from build123d import *

# Parameters (mm, degrees)
SKETCH_1_W             = 95
SKETCH_1_H             = 95
EXTRUDE_1_DEPTH        = 2
SKETCH_2_W             = 95
SKETCH_2_H             = 2
EXTRUDE_2_DEPTH        = 10
FILLET_1_R             = 20
SKETCH_3_W             = 60
SKETCH_3_H             = 10
CUT_EXTRUDE_1_DEPTH    = 106.115412761
EXTRUDE_START          = 33
EXTRUDE_3_DEPTH        = 1
PATTERN_LINEAR_1_COUNT = 2
PATTERN_LINEAR_1_PITCH = 12
MIRROR_START           = 33
MIRROR_1_COPY_1_DEPTH  = 1
SKETCH_7_R             = 1.5
CUT_EXTRUDE_2_DEPTH    = 2


with BuildPart() as part:
    # 草图1 → 凸台-拉伸1 (new body)
    with BuildSketch(Plane.XY):
        Rectangle(SKETCH_1_W, SKETCH_1_H)
    extrude(amount=EXTRUDE_1_DEPTH)

    # 草图2 → 凸台-拉伸2 (add)
    with BuildSketch(Plane.XY.offset(2)):
        with Locations((0, -46.5)):
            Rectangle(SKETCH_2_W, SKETCH_2_H)
    extrude(amount=EXTRUDE_2_DEPTH)

    # 圆角1
    fillet_1_edges = [part.edges().sort_by_distance(p)[0] for p in [
        (-47.5, 47.5, 1),
        (47.5, 47.5, 1),
    ]]
    fillet(fillet_1_edges, radius=FILLET_1_R)

    # 草图3 → 切除-拉伸1 (cut, through all)
    with BuildSketch(Plane(origin=(0, -45.5, 0), x_dir=(1, 0, 0), z_dir=(0, 1, 0))):
        with Locations((0, -7)):
            Rectangle(SKETCH_3_W, SKETCH_3_H)
    extrude(amount=-CUT_EXTRUDE_1_DEPTH, mode=Mode.SUBTRACT)

    # 草图5 → 凸台-拉伸3 (add, symmetric)
    with BuildSketch(Plane(origin=(0, 0, 0), x_dir=(0, 0, -1), z_dir=(1, 0, 0)).offset(EXTRUDE_START)):
        Polygon((-1.499876111, -46.213636553), (-1.499876111, -21.213636553), (-10.151701689, -46.213636553), align=None)
    extrude_3 = extrude(amount=EXTRUDE_3_DEPTH, both=True)

    # 阵列(线性)1: 凸台-拉伸3 ×2
    with Locations(*[(i * PATTERN_LINEAR_1_PITCH, 0, 0) for i in range(1, PATTERN_LINEAR_1_COUNT)]):
        add(extrude_3)

    # 镜向1: 凸台-拉伸3 across plane
    add(extrude_3.mirror(Plane(origin=(0, 0, 0), x_dir=(0, 0, 1), z_dir=(1, 0, 0))))

    # 镜向1 copy 1 sketch → 镜向1 copy 1 (add, symmetric)
    with BuildSketch(Plane(origin=(-12, 0, 0), x_dir=(0, 0, -1), z_dir=(-1, 0, 0)).offset(MIRROR_START)):
        Polygon((-1.499876111, 46.213636553), (-1.499876111, 21.213636553), (-10.151701689, 46.213636553), align=None)
    extrude(amount=MIRROR_1_COPY_1_DEPTH, both=True)

    # 草图7 → 切除-拉伸2 (cut)
    with BuildSketch(Plane(origin=(0, -45.5, 0), x_dir=(1, 0, 0), z_dir=(0, 1, 0))):
        with Locations(Location((-39, -7, 0), (0, 0, 270))):
            Circle(SKETCH_7_R)
        with Locations(Location((39, -7, 0), (0, 0, 90))):
            Circle(SKETCH_7_R)
    extrude(amount=-CUT_EXTRUDE_2_DEPTH, mode=Mode.SUBTRACT)


solid = part.part
Source: CAD feature listing. Evaluate the final solid. Frame: model axes, mm. A direction names the side the tool comes from. Round coordinates to 2 decimals unless told otherwise and drop trailing zeros. Loops run counter-clockwise (first coordinate to the right, second up) from the corner with the lowest first, then second, coordinate; pieces in that order, holes last.
Q1. Mould query, pull axis X, two halves, no side actions, for faces 1 (the face through (34, -39, 4)), 2 (the face through (-44, -37, 5)), 3 (the face through (47.5, -15.7, 1.5)), 4 (the face through (-33.014, -33.919, 5.897)). Classes: pulls with the +X half, pulls with the -X half, needs draft (parallel to the pull), parting line crosses it, or undercut.
Q2. First-contact query: P1, Ø2, axis at x = 35, y = 36, coming from the +Z side; P2, Ø6.5, axis at y = -32.5, z = 5.5, coming from the -X side; P3, Ø3, axis at x = 39, z = 6.5, coming from the +Y side. Flat tips, straight axial feed; report the tip coordinate or a pass-through.
Q3. Access query for faces 5 (the face through (46, -39, 4)), 6 (the face through (40.464, -46.486, 7.325)), 7 (the face through (-37, -45.5, 7)), 8 (the face through (-41.797, 41.486, 1.014)), 9 (the face through (-46, -37, 5)). Directions: +Z, -Z, +X, -X, +Y, -Y. A direction counts if a zero-diameter tool reaches every point of the face in a straight line with its end or side. Return the directions, or none.
Q4. Section C-C, the plane y = -4. Return loops of the section in (x, z).
Q5. Section A-A, the plane x = 39. Return loops of the section in (y, z).
Q6. Section B-B, the plane z = 7. State how many separate pieces and enclosed holes the cut face has, plus the area to 3 significant figures.
Q7. Ray query, line 1 (X direction, y = -46.2, z = 7); line 2 (X direction, y = -43, z = 7.25); line 3 (Z direction, x = 39, y = -46). Return the intervals inside material, ascending.
Solutions:
1. face 1: undercut
1. face 2: undercut
1. face 3: pulls with the +X half
1. face 4: needs draft
2. P1: stops at z = 2
2. P2: stops at x = -46
2. P3: stops at y = -45.5
3. face 5: +Z, +X, +Y
3. face 6: +Y, -Y
3. face 7: +Z, +Y
3. face 8: +Z, -Z, -X, +Y
3. face 9: +Z, -X, +Y
4. outline: (-47.5, 0) - (47.5, 0) - (47.5, 2) - (-47.5, 2) - close
5. outline: (-47.5, 0) - (43.86, 0) - (43.86, 2) - (-45.5, 2) - (-45.5, 5.5) - (-47.5, 5.5) - close; (-47.5, 8.5) - (-45.5, 8.5) - (-45.5, 12) - (-47.5, 12) - close
6. separate pieces: 4
6. enclosed holes: 0
6. area: 125 mm2
7. line 1: x = -47.5 to -40.5, -37.5 to -30, 30 to 37.5, 40.5 to 47.5
7. line 2: x = -46 to -44, -34 to -32, 32 to 34, 44 to 46
7. line 3: z = 0 to 5.5, 8.5 to 12
